Design review of the part built by this model. Coordinates are the model's own, in mm. A direction names the side the tool comes from. Give positions to 0.01 mm unless a question says otherwise; leave off trailing zeros. Order: outer loops, then holes, each group sorted by start corner. A loop starts at its lowest first (then second) coordinate and runs counter-clockwise, first axis right, second up. Notation, with made-up numbers: (-3.75, 18) -> (45.25, 18) arc R32 ccw to (45.25, 55) -> close; hole circle Ø5 at (-0.5, 24.25). An arc over 180 degrees is marked (long way). One line per item, written item: value. Start each with the question number.
1) Consider section D-D (z = 2.25). State the section outline as (x, y) points.
2) Tool access review of faces 4 (the face through (3, 5, 0)), 5 (the face through (-3, 10, 0)), 6 (the face through (-3, 3.5, 1.8)): name each direction out of +Z, -Z, +X, -X, +Y, -Y from which nothing blocks a thin tool from reaching the whole face with its end or side.
3) Consider section A-A (x = 0). State the section outline as (y, z) points.
4) Consider section B-B (y = 4.25). State the section outline as (x, z) points.
5) Wall thickness on line 1 along Z through (x, y) = (0, 8.25); line 2 along Z through (x, y) = (0, 4.5); line 3 along Y through (x, z) = (0, 2.25): over which ranges is each line inside the solid? List them lowest first. Write a range as from..to.
6) For pin 1 (2 mm diameter, centred on y = 5.5, z = 2, fed in from -X), flat-tipped, find the tip position at first contact; note if it passes through.
7) Consider section C-C (x = -2.25). State the section outline as (y, z) points.
8) The part is to be moulded in two halves that separate along Y. For faces 1 (the face through (2, 2, 1)), 2 (the face through (3, 3.5, -1.8)), 3 (the face through (-0.54, 5.76, 2.44)), say which applies: released by +Y, released by -Y, zero draft, split by the parting line, or undercut.
Autodesk Inventor part; units mm, degrees
ref_plane "YZ Plane" through (0, 0, 0) normal (1, 0, 0) x (0, 1, 0)
ref_plane "XZ Plane" through (0, 0, 0) normal (0, 1, 0) x (-1, 0, 0)
ref_plane "XY Plane" through (0, 0, 0) normal (0, 0, 1) x (1, 0, 0)
sketch "Sketch1" plane through (0, 0, 0) normal (0, 0, 1) x (1, 0, 0)
  line L0 (0, 0) -> (0.5, 0)
  line L1 (0.5, 0) -> (1.9004, 2)
  line L2 (1.9004, 2) -> (4.5, 2)
  line L3 (4.5, 2) -> (4.5, 5)
  line L4 (4.5, 5) -> (2.5, 5)
  line L5 (2.5, 5) -> (2.5, 6.5)
  line L6 (2.5, 6.5) -> (3, 6.5)
  line L7 (3, 6.5) -> (3, 12.5)
  line L8 (3, 12.5) -> (0, 12.5)
  line L9 (0, 12.5) -> (0, 0)
  dimension "d0" = 0.5
  dimension "d1" = 125
  dimension "d3" = 4.5
  dimension "d4" = 3
  dimension "d5" = 2.5
  dimension "d6" = 1.5
  dimension "d7" = 3
  dimension "d8" = 10.5
  dimension "d9" = 12.5
revolve "Revolution1" add sketch "Sketch1" angle 360 about axis through (0, 12.5, 0) along (0, -1, 0)
sketch "Sketch2" plane through (0, 5, 0) normal (0, 1, 0) x (1, 0, 0)
  circle A0 centre (0, 0) radius 4.5
  line L0 (4.0415, 0) -> (2.0207, -3.5)
  line L1 (2.0207, -3.5) -> (-2.0207, -3.5)
  line L2 (-2.0207, -3.5) -> (-4.0415, 0)
  line L3 (-4.0415, 0) -> (-2.0207, 3.5)
  line L4 (-2.0207, 3.5) -> (2.0207, 3.5)
  line L5 (2.0207, 3.5) -> (4.0415, 0)
  dimension "d11" = 7
extrude "Extrusion1" cut sketch "Sketch2" against normal up to surface (3 mm away)
thread "Thread1"
sketch "Sketch3" plane through (0, 12.5, 0) normal (0, 1, 0) x (1, 0, 0)
  circle A0 centre (0, 0) radius 3
  circle A1 centre (0, 0) radius 1
  dimension "d16" = 2
extrude "Extrusion2" cut sketch "Sketch3" against normal blind 10.5 contours A1
sketch "Sketch4" plane through (0, 0, 0) normal (0, -1, 0) x (1, 0, 0)
  circle A0 centre (0, 0) radius 0.5
  circle A1 centre (0, 0) radius 0.2
  dimension "d19" = 0.4
extrude "Extrusion3" cut sketch "Sketch4" against normal up to surface (2 mm away) contours A1
properties part number "ChimeraNozzle.4" material "Brass, Soft Yellow"
Checked values:
1. outline: (-2.74, 2) -> (2.74, 2) -> (2.74, 5) -> (1.09, 5) -> (1.09, 6.5) -> (1.98, 6.5) -> (1.98, 12.5) -> (-1.98, 12.5) -> (-1.98, 6.5) -> (-1.09, 6.5) -> (-1.09, 5) -> (-2.74, 5) -> close
2. face 4: none
2. face 5: +Y
2. face 6: +Z, -X, +Y, -Y
3. outline: (0, -0.5) -> (2, -1.9) -> (2, -3.5) -> (5, -3.5) -> (5, -2.5) -> (6.5, -2.5) -> (6.5, -3) -> (12.5, -3) -> (12.5, -1) -> (2, -1) -> (2, -0.2) -> (0, -0.2) -> close; (0, 0.2) -> (2, 0.2) -> (2, 1) -> (12.5, 1) -> (12.5, 3) -> (6.5, 3) -> (6.5, 2.5) -> (5, 2.5) -> (5, 3.5) -> (2, 3.5) -> (2, 1.9) -> (0, 0.5) -> close
4. outline: (-4.04, 0) -> (-2.02, -3.5) -> (2.02, -3.5) -> (4.04, 0) -> (2.02, 3.5) -> (-2.02, 3.5) -> close; hole circle Ø2 at (0, 0)
5. line 1: z = -3..-1, 1..3
5. line 2: z = -3.5..-1, 1..3.5
5. line 3: y = 2..12.5
6. pin 1: stops at x = -3.39
7. outline: (2, -3.1) -> (5, -3.1) -> (5, -1.09) -> (6.5, -1.09) -> (6.5, -1.98) -> (12.5, -1.98) -> (12.5, 1.98) -> (6.5, 1.98) -> (6.5, 1.09) -> (5, 1.09) -> (5, 3.1) -> (2, 3.1) -> close
8. face 1: released by -Y
8. face 2: zero draft
8. face 3: undercut
